The listing builds one solid part. Answer for the finished solid, in the listing's coordinates (mm). Face numbers are marked on the shaded views. A direction names the side the tool comes from. Round coordinates to 2 decimals unless told otherwise and drop trailing zeros. Write each loop counter-clockwise with the first axis right and the second up, starting at its lowest first coordinate (ties: lowest second). Pieces come first, ordered by that corner, then holes.
(1) For the marked faces 4, 5, 6 and 7, determine the directions among +Z, -Z, +X, -X, +Y, -Y from which every point of the face is accessible in a straight line to the end or side of a thin tool.
(2) A cutting plane is placed at A-A, the plane y = -12.5. Give the vertices of the cut face in (x, z).
(3) Each of these flat-tipped pins is pushed along its axis until it touches: pin 1 Ø10 at (x, y) = (-26.5, 49) entering from -Z; pin 2 Ø8 at (x, y) = (-16, 41.5) entering from -Z; pin 3 Ø6 at (x, y) = (29, 28.5) entering from -Z. Where does it stop, or does it pass through?
(4) The mould has two halves that part along Z. Classify the marked faces 1, 2 and 3: +Z half, -Z half, draft (parallel to the pull), parting line (faces both ways), or undercut.
(5) A cutting plane is placed at C-C, the plane y = 39. Give the vertices of the cut face in (x, z).
(6) A cutting plane is placed at B-B, the plane z = 0. Give the vertices of the cut face in (x, y), and give its area (3 significant figures).
(7) Find the intervals of material crossed by probe 1 along X at (y, z) = (-5, 0); probe 2 along Z at (x, y) = (0, 29.5); probe 3 along X at (y, z) = (-9.5, -29.5), in increasing order.
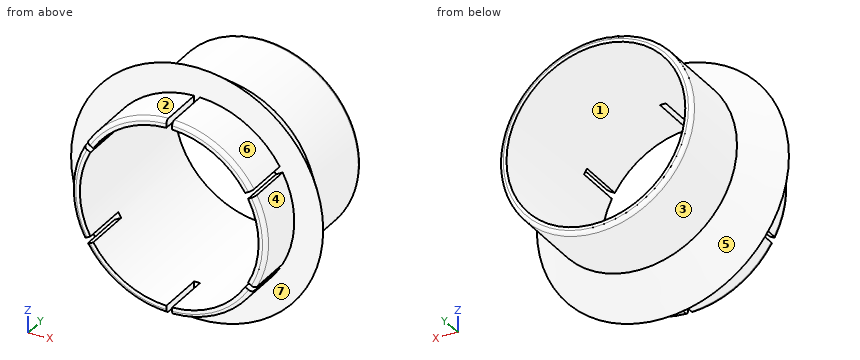
Autodesk Inventor part; units mm, degrees
ref_plane "YZ Plane" through (0, 0, 0) normal (1, 0, 0) x (0, 1, 0)
ref_plane "XZ Plane" through (0, 0, 0) normal (0, 1, 0) x (-1, 0, 0)
ref_plane "XY Plane" through (0, 0, 0) normal (0, 0, 1) x (1, 0, 0)
sketch "Sketch1" plane through (0, 0, 0) normal (0, 0, 1) x (1, 0, 0)
  line L0 (-50.35, 0) -> (-46.35, 0)
  line L1 (-46.35, 0) -> (-46.35, -25)
  line L2 (-46.35, -25) -> (-48.35, -25)
  line L3 (-50.35, -23) -> (-50.35, 0)
  line L4 (-46.35, 20) -> (-50, 20)
  line L5 (-50, 20) -> (-50, 58)
  line L6 (-48, 60) -> (-46.35, 60)
  line L7 (-46.35, 60) -> (-46.35, 20)
  line L8 (-50.35, 0) -> (-65.35, 0)
  line L9 (-65.35, 0) -> (-50, 20)
  line L10 (-46.35, 20) -> (-46.35, 0)
  arc A0 (-48, 60) -> (-50, 58) centre (-48, 58) ccw
  arc A1 (-50.35, -23) -> (-48.35, -25) centre (-48.35, -23) ccw
  line L11 (0, -42.5799) -> (0, 77.5799)
  point P0 (0, 0)
  point P1 (-50.35, -25)
  point P2 (-50, 60)
  point P3 (-48.35, 0)
  dimension "d4" = 4
  dimension "d5" = 25
  dimension "d7" = 40
  dimension "d8" = 15
  dimension "d9" = 50.35
  dimension "d10" = 2
  dimension "d12" = 20
  dimension "d20" = 50
revolve "Revolution1" add sketch "Sketch1" angle 360 about axis through (0, -10, 0) along (0, 1, 0)
sketch "Sketch2" plane through (0, -25, 0) normal (0, -1, 0) x (1, 0, 0)
  line L0 (1.5, 41.35) -> (-1.5, 41.35)
  line L1 (-1.5, 41.35) -> (-1.5, 51.35)
  line L2 (-1.5, 51.35) -> (1.5, 51.35)
  line L3 (1.5, 51.35) -> (1.5, 41.35)
  circle A0 centre (0, 0) radius 46.35
  line L4 (1.5, 41.35) -> (-1.5, 51.35) construction
  line L5 (-1.5, 41.35) -> (1.5, 51.35) construction
  point P0 (0, 46.35)
  dimension "d13" = 3
  dimension "d14" = 10
extrude "Extrusion1" cut sketch "Sketch2" against normal blind 25 contours L0 L1 A0 L3 | A0 L1 L2 L3 picked at (-0.1667, 43.0158)
pattern_circular "Circular Pattern1" count 6 over 360 about axis through (0, -10, 0) along (0, 1, 0) of "Extrusion1"
properties part number "top-ventilation-tube-adapter-100.9mmID-to-95mmID"
Solutions:
1. face 4: +X, -Y
1. face 5: +Y
1. face 6: +Z, +X, -Y
1. face 7: -Y
2. outline: (-44.34, -23.86) - (-40.87, -21.86) arc R46.35 cw to (-40.87, 21.86) - (-44.34, 23.86) arc R50.35 ccw to start; (-42.84, -26.46) arc R50.35 ccw to (-1.5, -50.33) - (-1.5, -46.33) arc R46.35 cw to (-39.37, -24.46) - close; (-42.84, 26.46) - (-39.37, 24.46) arc R46.35 cw to (-1.5, 46.33) - (-1.5, 50.33) arc R50.35 ccw to start; (1.5, -50.33) arc R50.35 ccw to (42.84, -26.46) - (39.37, -24.46) arc R46.35 cw to (1.5, -46.33) - close; (1.5, 46.33) arc R46.35 cw to (39.37, 24.46) - (42.84, 26.46) arc R50.35 ccw to (1.5, 50.33) - close; (40.87, -21.86) - (44.34, -23.86) arc R50.35 ccw to (44.34, 23.86) - (40.87, 21.86) arc R46.35 cw to start
3. pin 1: stops at z = -45.14
3. pin 2: stops at z = -48.54
3. pin 3: stops at z = -42.71
4. face 1: undercut
4. face 2: +Z half
4. face 3: parting line
5. outline: circle Ø100 at (0, 0); hole circle Ø92.7 at (0, 0)
6. outline: (-65.35, 0) - (-50.35, 0) - (-50.35, -23) arc R2 ccw to (-48.35, -25) - (-46.35, -25) - (-46.35, 60) - (-48, 60) arc R2 ccw to (-50, 58) - (-50, 20) - close; (46.35, -25) - (48.35, -25) arc R2 ccw to (50.35, -23) - (50.35, 0) - (65.35, 0) - (50, 20) - (50, 58) arc R2 ccw to (48, 60) - (46.35, 60) - close
6. area: 942 mm2
7. probe 1: x = -50.35 to -46.35, 46.35 to 50.35
7. probe 2: z = -50 to -46.35, 46.35 to 50
7. probe 3: x = -40.8 to -35.75, 35.75 to 40.8
